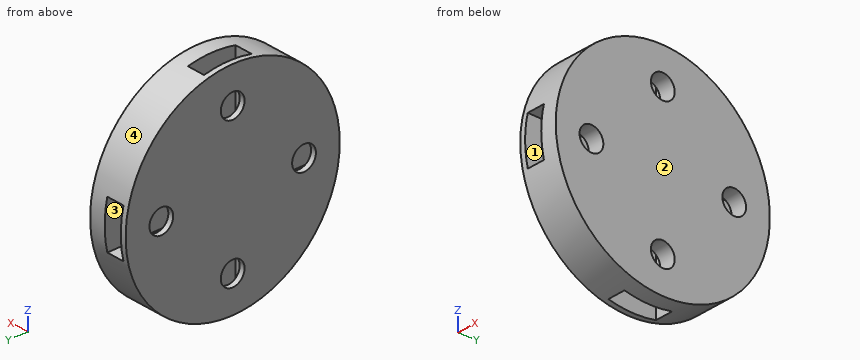
from build123d import *

# Parameters (mm, degrees)
BOX043_W                    = 6
BOX043_H                    = 4
BOX043_DEPTH                = 1.5
BOX046_W                    = 6
BOX046_H                    = 4
BOX046_DEPTH                = 1.5
BOX045_W                    = 6
BOX045_H                    = 4
BOX045_DEPTH                = 1.5
BOX044_W                    = 6
BOX044_H                    = 4
BOX044_DEPTH                = 1.5
COMPOUND834_ROLL_ANGLE      = 90
COMPOUND834_PLACEMENT_ANGLE = -90
CYLINDER496_R               = 1
CYLINDER496_DEPTH           = 10
CYLINDER497_R               = 1
CYLINDER497_DEPTH           = 10
CYLINDER495_R               = 1
CYLINDER495_DEPTH           = 10
CYLINDER494_R               = 1
CYLINDER494_DEPTH           = 10
COMPOUND833_ROLL_ANGLE      = 90
COMPOUND833_PLACEMENT_ANGLE = -90
CYLINDER493_R               = 9
CYLINDER493_DEPTH           = 3.3


with BuildPart() as krychle043:
    # Box043 → Box043 (new body)
    with BuildSketch(Plane(origin=(2, 3, -9.4), x_dir=(0, 1, 0), z_dir=(0, 0, 1))):
        with Locations((3, 2)):
            Rectangle(BOX043_W, BOX043_H)
    extrude(amount=BOX043_DEPTH)


with BuildPart() as krychle046:
    # Box046 → Box046 (new body)
    with BuildSketch(Plane(origin=(-3, 2, -9.4), x_dir=(-1, 0, 0), z_dir=(0, 0, 1))):
        with Locations((3, 2)):
            Rectangle(BOX046_W, BOX046_H)
    extrude(amount=BOX046_DEPTH)


with BuildPart() as krychle045:
    # Box045 → Box045 (new body)
    with BuildSketch(Plane(origin=(-2, -3, -9.4), x_dir=(0, -1, 0), z_dir=(0, 0, 1))):
        with Locations((3, 2)):
            Rectangle(BOX045_W, BOX045_H)
    extrude(amount=BOX045_DEPTH)


with BuildPart() as compound834:
    # Box044 → Box044 (new body)
    with BuildSketch(Plane(origin=(3, -2, -9.4), x_dir=(1, 0, 0), z_dir=(0, 0, 1))):
        with Locations((3, 2)):
            Rectangle(BOX044_W, BOX044_H)
    extrude(amount=BOX044_DEPTH)

    # Compound834: union Krychle043, Krychle046, Krychle045
    add(krychle043.part)
    add(krychle046.part)
    add(krychle045.part)


with BuildPart() as compound834_1:
    # Compound834 roll: moved
    add(compound834.part.rotate(Axis((0, 0, 0), (1, 0, 0)), COMPOUND834_ROLL_ANGLE))


with BuildPart() as compound834_2:
    # Compound834 placement: moved
    add(compound834_1.part.moved(Location((6, 0, 60))).rotate(Axis((6, 0, 60), (0, 0, 1)), COMPOUND834_PLACEMENT_ANGLE))


with BuildPart() as obj1:
    # Cylinder496 → Cylinder496 (new body)
    with BuildSketch(Plane(origin=(0, 6, -9.6), x_dir=(0, 1, 0), z_dir=(0, 0, 1))):
        Circle(CYLINDER496_R)
    extrude(amount=CYLINDER496_DEPTH)


with BuildPart() as obj2:
    # Cylinder497 → Cylinder497 (new body)
    with BuildSketch(Plane(origin=(-6, 0, -9.6), x_dir=(-1, 0, 0), z_dir=(0, 0, 1))):
        Circle(CYLINDER497_R)
    extrude(amount=CYLINDER497_DEPTH)


with BuildPart() as obj3:
    # Cylinder495 → Cylinder495 (new body)
    with BuildSketch(Plane(origin=(0, -6, -9.6), x_dir=(0, -1, 0), z_dir=(0, 0, 1))):
        Circle(CYLINDER495_R)
    extrude(amount=CYLINDER495_DEPTH)


with BuildPart() as compound833:
    # Cylinder494 → Cylinder494 (new body)
    with BuildSketch(Plane(origin=(6, 0, -9.6), x_dir=(1, 0, 0), z_dir=(0, 0, 1))):
        Circle(CYLINDER494_R)
    extrude(amount=CYLINDER494_DEPTH)

    # Compound833: union obj1, obj2, obj3
    add(obj1.part)
    add(obj2.part)
    add(obj3.part)


with BuildPart() as compound833_1:
    # Compound833 roll: moved
    add(compound833.part.rotate(Axis((0, 0, 0), (1, 0, 0)), COMPOUND833_ROLL_ANGLE))


with BuildPart() as compound833_2:
    # Compound833 placement: moved
    add(compound833_1.part.moved(Location((13.85, 0, 60))).rotate(Axis((13.85, 0, 60), (0, 0, 1)), COMPOUND833_PLACEMENT_ANGLE))


with BuildPart() as cut657:
    # Cylinder493 → Cylinder493 (new body)
    with BuildSketch(Plane(origin=(16.75, 0, 60), x_dir=(0, -1, 0), z_dir=(-1, 0, 0))):
        Circle(CYLINDER493_R)
    extrude(amount=CYLINDER493_DEPTH)

    # Cut656: cut Compound833
    add(compound833_2.part, mode=Mode.SUBTRACT)

    # Cut657: cut Compound834
    add(compound834_2.part, mode=Mode.SUBTRACT)


solid = cut657.part
CAD build for the part. Positions are in the model's coordinates, mm. Face numbers are marked on the shaded views. Give positions to 0.01 mm unless a question says otherwise; leave off trailing zeros. Loops run counter-clockwise (first coordinate to the right, second up) from the corner with the lowest first, then second, coordinate; pieces in that order, holes last. Notation, with made-up numbers: M -13.5,12.5 L 8.5,12.5 A21 ccw 8.5,25.5 Z; hole C -34,15 d6. An arc over 180 degrees is marked long. Write each question's results on one line, items separated by ' | '.
Q1. Flat gauge pins, fed straight in: P1, Ø1.5, axis at x = 15.5, y = -1, coming from the +Z side; P2, Ø1.2, axis at x = 15, z = 66, coming from the +Y side; P3, Ø3, axis at y = 0, z = 54, coming from the -X side; P4, Ø1.2, axis at x = 15, y = -5.5, coming from the -Z side. Where does each tip first touch, or does it go through?
Geometry check:
P1: stops at z = 69 | P2: stops at y = 7.2 | P3: stops at x = 13.45 | P4: stops at z = 52.45
Q2. Band-saw the part on A-A on y = 0. Write the cut outline in (x, z).
Geometry check:
outline: M 13.45,51 L 13.9,51 L 13.9,53 L 13.45,53 Z; M 13.45,55 L 13.9,55 L 13.9,57 L 15.4,57 L 15.4,55 L 16.75,55 L 16.75,65 L 15.4,65 L 15.4,63 L 13.9,63 L 13.9,65 L 13.45,65 Z; M 13.45,67 L 13.9,67 L 13.9,69 L 13.45,69 Z; M 15.4,51 L 16.75,51 L 16.75,53 L 15.4,53 Z; M 15.4,67 L 16.75,67 L 16.75,69 L 15.4,69 Z
Q3. Mould opens along Z. For the marked faces 1, 2, 3 and 4 say: pulls with the +Z half, pulls with the -Z half, needs draft (parallel to the pull), parting line crosses it, or undercut.
Geometry check:
face 1: undercut | face 2: needs draft | face 3: undercut | face 4: parting line crosses it
Q4. Band-saw the part on D-D on x = 16.05. Write the cut outline in (y, z).
Geometry check:
outline: C 0,60 d18; hole C -6,60 d2; hole C 0,54 d2; hole C 0,66 d2; hole C 6,60 d2
Q5. Band-saw the part on B-B on z = 60. Write the cut outline in (x, y), and give its area (3 significant figures).
Geometry check:
outline: M 13.45,-9 L 13.9,-9 L 13.9,-7 L 13.45,-7 Z; M 13.45,-5 L 13.9,-5 L 13.9,-3 L 15.4,-3 L 15.4,-5 L 16.75,-5 L 16.75,5 L 15.4,5 L 15.4,3 L 13.9,3 L 13.9,5 L 13.45,5 Z; M 13.45,7 L 13.9,7 L 13.9,9 L 13.45,9 Z; M 15.4,-9 L 16.75,-9 L 16.75,-7 L 15.4,-7 Z; M 15.4,7 L 16.75,7 L 16.75,9 L 15.4,9 Z | area: 34.2 mm²
Q6. Probe probe 1 along X at (y, z) = (-7, 61); probe 2 along Y at (x, z) = (13.65, 59.5); probe 3 along Z at (x, y) = (15, 6.5). List the from-to ranges inside material, lowest first.
Geometry check:
probe 1: x = 13.45 to 13.9, 15.4 to 16.75 | probe 2: y = -8.99 to -6.87, -5.13 to 5.13, 6.87 to 8.99 | probe 3: z = 53.78 to 58, 62 to 66.22
Q7. Band-saw the part on C-C on y = -5.75. Write the cut outline in (x, z).
Geometry check:
outline: M 13.45,53.08 L 16.75,53.08 L 16.75,59.03 L 15.4,59.03 L 15.4,58 L 13.9,58 L 13.9,59.03 L 13.45,59.03 Z; M 13.45,60.97 L 13.9,60.97 L 13.9,62 L 15.4,62 L 15.4,60.97 L 16.75,60.97 L 16.75,66.92 L 13.45,66.92 Z
